Geometry: final body of the model. Coordinates: model frame, mm. Give positions to 0.01 mm unless a question says otherwise; leave off trailing zeros. Write each loop counter-clockwise with the first axis right and the second up, starting at its lowest first coordinate (ties: lowest second). Pieces come first, ordered by that corner, then holes. Notation, with made-up numbers: M 60,66.5 L 118,66.5 A10 ccw 118,73.5 Z; hole C -14.5,5.5 d8. An arc over 180 degrees is marked long. Use a Markdown table: item, result. Add a question column.
(1) Material intervals for L1, parallel to X at y = 0, z = 3.75; L2, parallel to X at y = -0.5, z = 13.25; L3, parallel to Y at x = 0, z = 3, sorted ascending.
(2) Pin query (flat end, axial travel): pin 1 Ø5 at (x, z) = (3, 9) entering from +Y; pin 2 Ø3 at (y, z) = (-3, 15.5) entering from +X; pin 3 Ø4 at (x, z) = (-0.5, 11) entering from +Y. Return the tip coordinate at first contact, or that it passes through.
(3) Draft query along X for faces 1 (the flat face through (-3.3, -0.1, 0)), 2 (the cylindrical face through (-1.08, 4.88, 1.05)), 3 (the cylindrical face through (-3, 0, 4)). Return one class per face: released by +X, released by -X, zero draft, split by the parting line, or undercut.
(4) Cut plane A-A (z = 3.5). Output: boundary loops of the cut face in (x, y), plus the area to 3 significant figures.
```python
from build123d import *


with BuildPart() as f1:
    # F0 (on Front) → F1 (revolve)
    with BuildSketch(Plane.XZ):
        with BuildLine():
            Line((3, 0), (5, 0))
            Line((5, 0), (5, 2.066073))
            Line((5, 2.066073), (3.824242, 11.260495))
            ThreePointArc((3.824242, 11.260495), (3.052163, 12.696792), (2.659773, 14.279537))
            ThreePointArc((2.659773, 14.279537), (1.851925, 17.824059), (0, 20.952418))
            Line((0, 20.952418), (0, 17.068623))
            ThreePointArc((0, 17.068623), (0.450236, 15.609737), (0.667413, 14.09848))
            ThreePointArc((0.667413, 14.09848), (1.176377, 12.002533), (2.194559, 10.101127))
            ThreePointArc((2.194559, 10.101127), (2.79375, 8.903069), (3, 7.579501))
            Line((3, 7.579501), (3, 0))
        make_face()
    revolve(axis=Axis((0, 0, 16.671413), (0, 0, -1)))

    # F2 (on Front) → F3 (revolve, cut)
    with BuildSketch(Plane.XZ):
        Polygon((9.900054, 13.367673), (0, 21.913905), (0, 20.757873), (3.29275, 15.589049), (3.29275, 13.155878), (5.5244, 2.163447), align=None)
    revolve(axis=Axis((0, 0, 21.335889), (0, 0, -1)), mode=Mode.SUBTRACT)


solid = f1.part
```
Answer list:
| question | item | result |
|---|---|---|
| 1 | L1 | -4.78 to -3, 3 to 4.78 |
| 1 | L2 | -2.82 to -0.63, 0.63 to 2.82 |
| 1 | L3 | -4.88 to -3, 3 to 4.88 |
| 2 | pin 1 | y = 4.19 |
| 2 | pin 2 | x = 2.05 |
| 2 | pin 3 | y = 4.11 |
| 3 | face 1 | zero draft |
| 3 | face 2 | split by the parting line |
| 3 | face 3 | undercut |
| 4 | outline | C 0,0 d9.63; hole C 0,0 d6 |
| 4 | area | 44.6 mm² |
